Input: part model. Units: mm. Frame: model coordinates. Give positions to 0.01 mm unless a question says otherwise; leave off trailing zeros. Write each loop counter-clockwise with the first axis right and the second up, starting at its lowest first coordinate (ties: lowest second). Pieces come first, ordered by that corner, then holes. Notation, with made-up numbers: (26.25, 50) - (51.25, 50) arc R26 ccw to (51.25, 76) - close; hole circle Ø2 at (65.25, 70). An arc over 180 degrees is marked (long way). Answer as CSV lines item,"result". Start each with the question number.
from build123d import *

# Parameters (mm, degrees)
SKETCH_1_W        = 80
SKETCH_1_H        = 160
EXTRUDE_1_DEPTH   = 2
CHAMFER_1_SIZE    = 2
HOLE_WIZARD_M81_D = 9


with BuildPart() as part:
    # Эскиз1 → Бобышка-Вытянуть1 (new body)
    with BuildSketch(Plane.XY):
        Rectangle(SKETCH_1_W, SKETCH_1_H)
    extrude(amount=EXTRUDE_1_DEPTH)

    # Фаска1
    chamfer_1_edges = [part.edges().sort_by_distance(p)[0] for p in [
        (40, -80, 1),
        (-40, -80, 1),
        (-40, 80, 1),
        (40, 80, 1),
    ]]
    chamfer(chamfer_1_edges, length=CHAMFER_1_SIZE)

    # Отверстие с зазором M81 (through all)
    with Locations(Plane.XY.offset(2)):
        with Locations((-20, 20), (20, 20), (-20, -20), (20, -20), (-20, 60), (20, 60), (20, -60), (-20, -60)):
            Hole(HOLE_WIZARD_M81_D / 2)


solid = part.part
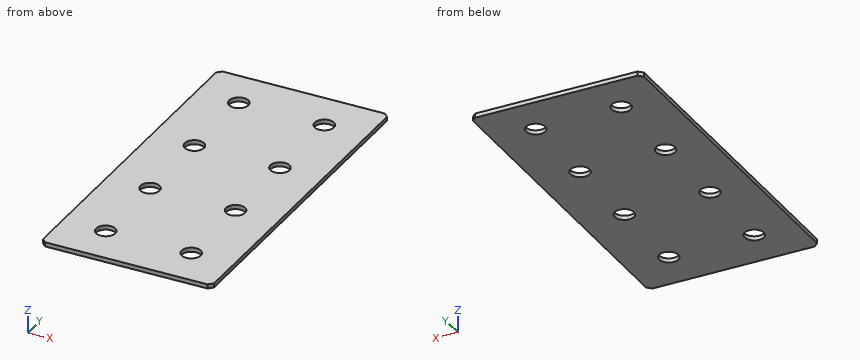
1) Material intervals for line 1 (Y direction, x = 20, z = 1); line 2 (X direction, y = 57.5, z = 1.45); line 3 (X direction, y = 16, z = 0.8), sorted ascending. Write a range as from..to.
2) Contact query for a flat-ended pin moving along its axis: P1, Ø5, axis at x = 15, y = -21.5, coming from the -Z side. Output: stop coordinate, or through.
3) Cut plane B-B on y = 20. Output: boundary loops of the cut face in (x, z), and give its area (3 significant figures).
4) Cut plane C-C on z = 1.55. State how many separate pieces and enclosed holes the cut face has, and give its area (3 significant figures).
5) Cut plane A-A on x = -20. Output: boundary loops of the cut face in (y, z).
Numbers:
1,line 1,"y = -80..-64.5, -55.5..-24.5, -15.5..15.5, 24.5..55.5, 64.5..80"
1,line 2,"x = -40..-23.74, -16.26..16.26, 23.74..40"
1,line 3,"x = -40..-22.06, -17.94..17.94, 22.06..40"
2,P1,"stops at z = 0"
3,outline,"(-40, 0) - (-24.5, 0) - (-24.5, 2) - (-40, 2) - close; (-15.5, 0) - (15.5, 0) - (15.5, 2) - (-15.5, 2) - close; (24.5, 0) - (40, 0) - (40, 2) - (24.5, 2) - close"
3,area,"124 mm²"
4,separate pieces,"1"
4,enclosed holes,"8"
4,area,"12,300 mm²"
5,outline,"(-80, 0) - (-64.5, 0) - (-64.5, 2) - (-80, 2) - close; (-55.5, 0) - (-24.5, 0) - (-24.5, 2) - (-55.5, 2) - close; (-15.5, 0) - (15.5, 0) - (15.5, 2) - (-15.5, 2) - close; (24.5, 0) - (55.5, 0) - (55.5, 2) - (24.5, 2) - close; (64.5, 0) - (80, 0) - (80, 2) - (64.5, 2) - close"
